Check sheet for the modelled part. Datum: model origin and axes. Units: mm. A direction names the side the tool comes from. Round coordinates to 2 decimals unless told otherwise and drop trailing zeros. Order: outer loops, then holes, each group sorted by start corner. A loop starts at its lowest first (then second) coordinate and runs counter-clockwise, first axis right, second up.
from build123d import *

# Parameters (mm, degrees)
BOSS_EXTRUDE1_DEPTH = 15.875
SKETCH5_W           = 3.175
SKETCH5_H           = 15.875
CUT_EXTRUDE1_DEPTH  = 3.175
SKETCH6_W           = 3.175
SKETCH6_H           = 15.875
CUT_EXTRUDE2_DEPTH  = 3.175
SKETCH7_W           = 19.05
SKETCH7_H           = 19.05
CUT_EXTRUDE4_DEPTH  = 10
SKETCH8_W           = 25
SKETCH8_H           = 7
CUT_EXTRUDE5_DEPTH  = 63.813266363
FILLET3_R           = 3
SKETCH2_W           = 25.4
SKETCH2_H           = 3.175
CUT_EXTRUDE6_DEPTH  = 4.175
SKETCH3_W           = 25.4
SKETCH3_H           = 3.175
CUT_EXTRUDE7_DEPTH  = 4.175
FILLET4_R           = 3


with BuildPart() as part:
    # Sketch1 → Boss-Extrude1 (new body)
    with BuildSketch(Plane(origin=(0, 0, 0), x_dir=(1, 0, 0), z_dir=(0, 1, 0))):
        with BuildLine():
            Line((-52.911658323, 34.190937018), (-2.431658323, 34.190937018))
            Line((-2.431658323, 34.190937018), (-2.431658323, -0.734062982))
            Line((-2.431658323, -0.734062982), (-52.911658323, -0.734062982))
            ThreePointArc((-52.911658323, -0.734062982), (-35.449158323, 16.728437018), (-52.911658323, 34.190937018))
        make_face()
    extrude(amount=BOSS_EXTRUDE1_DEPTH)

    # Sketch5 → Cut-Extrude1 (cut)
    with BuildSketch(Plane(origin=(0, 0, -34.190937018), x_dir=(-1, 0, 0), z_dir=(0, 0, -1))):
        with Locations((51.324158323, 7.9375)):
            Rectangle(SKETCH5_W, SKETCH5_H)
    extrude(amount=-CUT_EXTRUDE1_DEPTH, mode=Mode.SUBTRACT)

    # Sketch6 → Cut-Extrude2 (cut)
    with BuildSketch(Plane.XY.offset(0.734062982)):
        with Locations((-51.324158323, 7.9375)):
            Rectangle(SKETCH6_W, SKETCH6_H)
    extrude(amount=-CUT_EXTRUDE2_DEPTH, mode=Mode.SUBTRACT)

    # Sketch7 → Cut-Extrude4 (cut)
    with BuildSketch(Plane(origin=(0, 15.875, 0), x_dir=(1, 0, 0), z_dir=(0, 1, 0))):
        with Locations((-18.940408323, 16.728437018)):
            Rectangle(SKETCH7_W, SKETCH7_H)
    extrude(amount=-CUT_EXTRUDE4_DEPTH, mode=Mode.SUBTRACT)

    # Sketch8 → Cut-Extrude5 (cut, through all)
    with BuildSketch(Plane(origin=(0, 0, -34.190937018), x_dir=(-1, 0, 0), z_dir=(0, 0, -1))):
        with Locations((18.106658323, 7.9375)):
            Rectangle(SKETCH8_W, SKETCH8_H)
    extrude(amount=-CUT_EXTRUDE5_DEPTH, mode=Mode.SUBTRACT)

    # Fillet3
    # the kernel refuses this fillet: 3 mm, written as the material it takes off along each edge
    with BuildSketch(Plane(origin=(-57.236658323, 15.875, -34.190937018), x_dir=(0, 0, 1), z_dir=(1, 0, 0)), Plane(origin=(5.068341677, 15.875, 0.734062982), x_dir=(0, 0, -1), z_dir=(-1, 0, 0))) as fillet3_piece_1:
        with BuildLine():
            CenterArc((FILLET3_R, FILLET3_R), FILLET3_R, 180, 90)
            Line((0, FILLET3_R), (0, 0))
            Line((0, 0), (FILLET3_R, 0))
        make_face()
    extrude(amount=62.305, mode=Mode.SUBTRACT)
    with BuildSketch(Plane(origin=(-52.911658323, 15.875, -16.728437018), x_dir=(-0.24468593558499258, 0, 0.969602389088897), z_dir=(-0.969602389088897, 0, -0.24468593558499258))) as fillet3_piece_2:
        with BuildLine():
            CenterArc((17.4625 + FILLET3_R, -FILLET3_R), FILLET3_R, 90, 90)
            Line((17.4625 + FILLET3_R, 0), (17.4625, 0))
            Line((17.4625, 0), (17.4625, -FILLET3_R))
        make_face()
    revolve(axis=Axis((-52.911658323, 15.875, -16.728437018), (0, 1, 0)), revolution_arc=208.326548528, mode=Mode.SUBTRACT)

    # Sketch2 → Cut-Extrude6 (cut)
    with BuildSketch(Plane(origin=(0, 0, 0), x_dir=(-1, 0, 0), z_dir=(0, -1, 0))):
        with Locations((18.306658323, 26.253437018)):
            Rectangle(SKETCH2_W, SKETCH2_H)
    extrude(amount=-CUT_EXTRUDE6_DEPTH, mode=Mode.SUBTRACT)

    # Sketch3 → Cut-Extrude7 (cut)
    with BuildSketch(Plane(origin=(0, 0, 0), x_dir=(-1, 0, 0), z_dir=(0, -1, 0))):
        with Locations((18.306658323, 7.203437018)):
            Rectangle(SKETCH3_W, SKETCH3_H)
    extrude(amount=-CUT_EXTRUDE7_DEPTH, mode=Mode.SUBTRACT)

    # Fillet4
    fillet4_edges = [part.edges().sort_by_distance(p)[0] for p in [
        (-9.415408323, 15.875, -16.728437018),
        (-18.940408323, 15.875, -26.253437018),
        (-28.465408323, 15.875, -16.728437018),
        (-18.940408323, 15.875, -7.203437018),
    ]]
    fillet(fillet4_edges, radius=FILLET4_R)


solid = part.part
1) Sectioned sample at C-C on y = 1.75. Count the separate pieces of the cut face and the enclosed holes in it, and give its area (3 significant figures).
2) Set-up check for faces 1 (the face through (-5.607, 8, -17)), 2 (the face through (-5.607, 2, -26)), 3 (the face through (-28.465, 12, -17)): record each of +Z, -Z, +X, -X, +Y, -Y from which the full face is reachable in a straight line by a thin tool's end or side.
3) Gauge pin test, flat ends, axial feed: pin 1 (1.6 mm diameter, centred on y = 1.5, z = -7.5, fed in from -X); pin 2 (4 mm diameter, centred on y = 12.5, z = -11.5, fed in from -X); pin 3 (2 mm diameter, centred on y = 3.5, z = -30.5, fed in from -X). Record the tip position at first contact, or that the pin passes through.
4) Scan lines: line 1 (Z direction, x = -14, y = 2.5); line 2 (Z direction, x = -12.5, y = 12.5); line 3 (X direction, y = 2.75, z = -17). Record each from-to range of solid material in increasing order.
5) Sectioned sample at B-B on x = -25. Record the cut outline in (y, z) (1 decimal).
6) Draft check along Z on faces 4 (the face through (-26.42, 14.97, -33.34)), 5 (the face through (-18, 2, -24.666)), 6 (the face through (-18, 4.438, -17)). Enter one of: pulls with the +Z half, pulls with the -Z half, needs draft (parallel to the pull), parting line crosses it, or undercut.
Values found:
1. separate pieces: 1
1. enclosed holes: 2
1. area: 1,120 mm2
2. face 1: +Z, -Z
2. face 2: -Y
2. face 3: +Y
3. pin 1: stops at x = -38.62
3. pin 2: stops at x = -37.02
3. pin 3: stops at x = -43.6
4. line 1: z = -34.19 to -27.84, -24.67 to -8.79, -5.62 to 0.73
4. line 2: z = -34.19 to -26.25, -7.2 to 0.73
4. line 3: x = -35.45 to -2.43
5. outline: (0, -34.2) - (4.4, -34.2) - (4.4, 0.7) - (0, 0.7) - (0, -5.6) - (4.2, -5.6) - (4.2, -8.8) - (0, -8.8) - (0, -24.7) - (4.2, -24.7) - (4.2, -27.8) - (0, -27.8) - close; (11.4, -34.2) - (12.9, -34.2) arc R3 ccw to (15.9, -31.2) - (15.9, -29.3) arc R3 ccw to (12.9, -26.3) - (11.4, -26.3) - close; (11.4, -7.2) - (12.9, -7.2) arc R3 ccw to (15.9, -4.2) - (15.9, -2.3) arc R3 ccw to (12.9, 0.7) - (11.4, 0.7) - close
6. face 4: pulls with the -Z half
6. face 5: undercut
6. face 6: needs draft
